Check sheet for the modelled part. Datum: model origin and axes. Units: mm. Face numbers are marked on the shaded views. A direction names the side the tool comes from. Round coordinates to 2 decimals unless told otherwise and drop trailing zeros. Order: outer loops, then holes, each group sorted by start corner. A loop starts at its lowest first (then second) coordinate and runs counter-clockwise, first axis right, second up.
Q1. Cross-section at C-C on z = 12. Record the cut outline in (x, y) (1 decimal), then the cut area to 3 significant figures.
Q2. Cross-section at A-A on y = 1.5. Give the number of separate pieces and of enclosed holes in the cut face, then the cut area to 3 significant figures.
Q3. Scan lines: probe 1 along X at (y, z) = (2.5, 1); probe 2 along X at (y, z) = (16.5, 0) (1 decimal); probe 3 along Z at (x, y) = (-25, 7.5). Record each from-to range of solid material in increasing order.
Q4. Mould release check, pull along Z, two halves, no side actions. Record for the marked faces 1, 2 and 3: +Z half, -Z half, draft (parallel to the pull), parting line (faces both ways), or undercut.
Q5. Depth check by flat-ended pin: P1, Ø12.5, axis at x = 26.99, z = 26.99, coming from the +Y side (3 decimals); P2, Ø5, axis at x = 20.5, y = 14.5, coming from the +Z side; P3, Ø3, axis at x = -2, z = -31.5, coming from the +Y side (3 decimals); P4, Ø23, axis at x = 0, z = 0, coming from the -Y side. Enter the tip coordinate at first touch or a pass-through.
Q6. Set-up check for the marked faces 4, 5 and 6: record each of +Z, -Z, +X, -X, +Y, -Y from which the full face is reachable in a straight line by a thin tool's end or side.
Q7. Cross-section at B-B on x = 9.5. Record the cut outline in (y, z) (1 decimal).
from build123d import *

# Parameters (mm, degrees)
BOSS_EXTRUDE1_DEPTH                = 9.525
SKETCH2_R                          = 26.9875
CUT_EXTRUDE1_DEPTH                 = 3.175
SKETCH3_R                          = 26.9875
BOSS_EXTRUDE2_DEPTH                = 12.7
SKETCH4_R                          = 22.225
CUT_EXTRUDE2_DEPTH                 = 12.7
SKETCH5_R                          = 19.05
CUT_EXTRUDE3_DEPTH                 = 54.175326163
F_3_16_0_1875_DIAMETER_HOLE1_D     = 4.7625
F_3_16_0_1875_DIAMETER_HOLE1_DEPTH = 4.7625
F_3_16_0_1875_DIAMETER_HOLE1_TIP   = 1.430799349
BOSS_EXTRUDE3_DEPTH                = 6.35
FILLET1_R                          = 9.525
SKETCH10_R                         = 3.9751
CUT_EXTRUDE4_DEPTH                 = 55.021670999


with BuildPart() as part:
    # Sketch1 → Boss-Extrude1 (new body)
    with BuildSketch(Plane(origin=(0, 0, 0), x_dir=(1, 0, 0), z_dir=(0, 1, 0))):
        with BuildLine():
            Line((-26.9875, -36.5125), (26.9875, -36.5125))
            ThreePointArc((26.9875, -36.5125), (33.722692091, -33.722692091), (36.5125, -26.9875))
            Line((36.5125, -26.9875), (36.5125, 26.9875))
            ThreePointArc((36.5125, 26.9875), (33.722692091, 33.722692091), (26.9875, 36.5125))
            Line((26.9875, 36.5125), (-26.9875, 36.5125))
            ThreePointArc((-26.9875, 36.5125), (-33.722692091, 33.722692091), (-36.5125, 26.9875))
            Line((-36.5125, 26.9875), (-36.5125, -26.9875))
            ThreePointArc((-36.5125, -26.9875), (-33.722692091, -33.722692091), (-26.9875, -36.5125))
        make_face()
    extrude(amount=BOSS_EXTRUDE1_DEPTH)

    # Sketch2 → Cut-Extrude1 (cut)
    with BuildSketch(Plane.XZ):
        with Locations(Location((0, 0, 0), (0, 0, 270))):
            Circle(SKETCH2_R)
    extrude(amount=-CUT_EXTRUDE1_DEPTH, mode=Mode.SUBTRACT)

    # Sketch3 → Boss-Extrude2 (add)
    with BuildSketch(Plane(origin=(0, 9.525, 0), x_dir=(1, 0, 0), z_dir=(0, 1, 0))):
        with Locations(Location((0, 0, 0), (0, 0, 90))):
            Circle(SKETCH3_R)
    extrude(amount=BOSS_EXTRUDE2_DEPTH)

    # Sketch4 → Cut-Extrude2 (cut)
    with BuildSketch(Plane(origin=(0, 22.225, 0), x_dir=(1, 0, 0), z_dir=(0, 1, 0))):
        with Locations(Location((0, 0, 0), (0, 0, 270))):
            Circle(SKETCH4_R)
    extrude(amount=-CUT_EXTRUDE2_DEPTH, mode=Mode.SUBTRACT)

    # Sketch5 → Cut-Extrude3 (cut, through all)
    with BuildSketch(Plane(origin=(0, 9.525, 0), x_dir=(1, 0, 0), z_dir=(0, 1, 0))):
        with Locations(Location((0, 0, 0), (0, 0, 270))):
            Circle(SKETCH5_R)
    extrude(amount=-CUT_EXTRUDE3_DEPTH, mode=Mode.SUBTRACT)

    # 3/16 (0.1875) Diameter Hole1
    with Locations(Plane(origin=(0, 9.525, 0), x_dir=(1, 0, 0), z_dir=(0, 1, 0))):
        with Locations((0, 31.75)):
            Hole(F_3_16_0_1875_DIAMETER_HOLE1_D / 2, depth=F_3_16_0_1875_DIAMETER_HOLE1_DEPTH)
            with Locations((0, 0, -(F_3_16_0_1875_DIAMETER_HOLE1_DEPTH + F_3_16_0_1875_DIAMETER_HOLE1_TIP / 2))):  # 118° drill point
                Cone(0, F_3_16_0_1875_DIAMETER_HOLE1_D / 2, F_3_16_0_1875_DIAMETER_HOLE1_TIP, mode=Mode.SUBTRACT)

    # Sketch9 → Boss-Extrude3 (add)
    with BuildSketch(Plane(origin=(0, 9.525, 0), x_dir=(1, 0, 0), z_dir=(0, 1, 0))):
        with BuildLine():
            ThreePointArc((-24.590156824, 11.119772642), (-19.083044257, 19.083044257), (-11.119772642, 24.590156824))
            Line((-11.119772642, 24.590156824), (-20.252307909, 33.722692091))
            ThreePointArc((-20.252307909, 33.722692091), (-23.342440307, 35.787452547), (-26.9875, 36.5125))
            ThreePointArc((-26.9875, 36.5125), (-33.722692091, 33.722692091), (-36.5125, 26.9875))
            ThreePointArc((-36.5125, 26.9875), (-35.787452547, 23.342440307), (-33.722692091, 20.252307909))
            Line((-33.722692091, 20.252307909), (-24.590156824, 11.119772642))
        make_face()
        with BuildLine():
            ThreePointArc((11.119772642, 24.590156824), (19.083044257, 19.083044257), (24.590156824, 11.119772642))
            Line((24.590156824, 11.119772642), (33.722692091, 20.252307909))
            ThreePointArc((33.722692091, 20.252307909), (35.787452547, 23.342440307), (36.5125, 26.9875))
            ThreePointArc((36.5125, 26.9875), (33.722692091, 33.722692091), (26.9875, 36.5125))
            ThreePointArc((26.9875, 36.5125), (23.342440307, 35.787452547), (20.252307909, 33.722692091))
            Line((20.252307909, 33.722692091), (11.119772642, 24.590156824))
        make_face()
        with BuildLine():
            Line((33.722692091, -20.252307909), (24.590156824, -11.119772642))
            ThreePointArc((24.590156824, -11.119772642), (19.083044257, -19.083044257), (11.119772642, -24.590156824))
            Line((11.119772642, -24.590156824), (20.252307909, -33.722692091))
            ThreePointArc((20.252307909, -33.722692091), (23.342440307, -35.787452547), (26.9875, -36.5125))
            ThreePointArc((26.9875, -36.5125), (33.722692091, -33.722692091), (36.5125, -26.9875))
            ThreePointArc((36.5125, -26.9875), (35.787452547, -23.342440307), (33.722692091, -20.252307909))
        make_face()
        with BuildLine():
            Line((-20.252307909, -33.722692091), (-11.119772642, -24.590156824))
            ThreePointArc((-11.119772642, -24.590156824), (-19.083044257, -19.083044257), (-24.590156824, -11.119772642))
            Line((-24.590156824, -11.119772642), (-33.722692091, -20.252307909))
            ThreePointArc((-33.722692091, -20.252307909), (-35.787452547, -23.342440307), (-36.5125, -26.9875))
            ThreePointArc((-36.5125, -26.9875), (-33.722692091, -33.722692091), (-26.9875, -36.5125))
            ThreePointArc((-26.9875, -36.5125), (-23.342440307, -35.787452547), (-20.252307909, -33.722692091))
        make_face()
    extrude(amount=BOSS_EXTRUDE3_DEPTH)

    # Fillet1
    fillet1_edges = [part.edges().sort_by_distance(p)[0] for p in [
        (24.590156824, 12.7, 11.119772642),
        (11.119772642, 12.7, 24.590156824),
        (-11.119772642, 12.7, 24.590156824),
        (-24.590156824, 12.7, 11.119772642),
        (-11.119772642, 12.7, -24.590156824),
        (-24.590156824, 12.7, -11.119772642),
        (24.590156824, 12.7, -11.119772642),
        (11.119772642, 12.7, -24.590156824),
    ]]
    fillet(fillet1_edges, radius=FILLET1_R)

    # Sketch10 → Cut-Extrude4 (cut, through all)
    with BuildSketch(Plane(origin=(0, 15.875, 0), x_dir=(1, 0, 0), z_dir=(0, 1, 0))):
        with Locations(Location((-26.9875, 26.9875, 0), (0, 0, 270))):
            Circle(SKETCH10_R)
        with Locations(Location((26.9875, 26.9875, 0), (0, 0, 270))):
            Circle(SKETCH10_R)
        with Locations(Location((26.9875, -26.9875, 0), (0, 0, 270))):
            Circle(SKETCH10_R)
        with Locations(Location((-26.9875, -26.9875, 0), (0, 0, 270))):
            Circle(SKETCH10_R)
    extrude(amount=-CUT_EXTRUDE4_DEPTH, mode=Mode.SUBTRACT)


solid = part.part
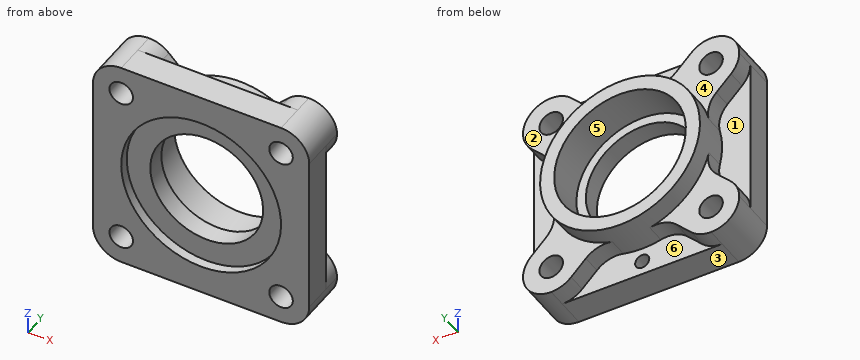
Results found:
1. outline: (-36.5, 0) - (-24.2, 0) - (-24.2, 3.2) - (-14.8, 3.2) - (-14.8, 9.5) - (-18.7, 9.5) - (-18.7, 22.2) - (-24.2, 22.2) - (-24.2, 15.9) - (-26.6, 15.9) - (-26.6, 9.5) - (-36.5, 9.5) - close; (14.8, 3.2) - (24.2, 3.2) - (24.2, 0) - (36.5, 0) - (36.5, 9.5) - (26.6, 9.5) - (26.6, 15.9) - (24.2, 15.9) - (24.2, 22.2) - (18.7, 22.2) - (18.7, 9.5) - (14.8, 9.5) - close
1. area: 524 mm2
2. separate pieces: 1
2. enclosed holes: 5
2. area: 2,770 mm2
3. probe 1: x = -36.51 to -26.97, 26.97 to 36.51
3. probe 2: x = -27 to -22.2, 22.2 to 27
3. probe 3: z = -36.51 to -30.43, -23.54 to 23.54, 30.43 to 36.51
4. face 1: undercut
4. face 2: draft
4. face 3: -Z half
5. P1: stops at y = 15.875
5. P2: stops at z = 35.64
5. P3: stops at y = 9.525
5. P4: passes through
6. face 4: +Z, -X, +Y
6. face 5: +Y
6. face 6: -Z, +Y
7. outline: (0, -36.5) - (9.5, -36.5) - (9.5, -26) - (15.9, -26) - (15.9, -25.3) - (22.2, -25.3) - (22.2, -20.1) - (9.5, -20.1) - (9.5, -16.5) - (3.2, -16.5) - (3.2, -25.3) - (0, -25.3) - close; (0, 25.3) - (3.2, 25.3) - (3.2, 16.5) - (9.5, 16.5) - (9.5, 20.1) - (22.2, 20.1) - (22.2, 25.3) - (15.9, 25.3) - (15.9, 26) - (9.5, 26) - (9.5, 36.5) - (0, 36.5) - close
